```python
from build123d import *

# Parameters (mm, degrees)
SKETCH1_R           = 6.35
BOSS_EXTRUDE1_DEPTH = 3.175
SKETCH2_W           = 5.08
SKETCH2_H           = 25.4
CUT_EXTRUDE1_DEPTH  = 7.35
SKETCH3_R           = 15.875
CUT_EXTRUDE2_DEPTH  = 7.35


with BuildPart() as part:
    # Sketch1 → Boss-Extrude1 (new body, symmetric)
    with BuildSketch(Plane.XY):
        with BuildLine():
            Line((-0.002676144, -12.7), (0.002676144, -12.7))
            Line((0.002676144, -12.7), (50.8, -12.7))
            ThreePointArc((50.8, -12.7), (71.550320151, -11.225320151), (73.025, 9.525))
            Line((73.025, 9.525), (73.025, 152.4))
            Line((73.025, 152.4), (-73.025, 152.4))
            Line((-73.025, 152.4), (-73.025, 9.525))
            ThreePointArc((-73.025, 9.525), (-71.550320151, -11.225320151), (-50.8, -12.7))
            Line((-50.8, -12.7), (-0.002676144, -12.7))
        make_face()
        with Locations((-60.325, 0)):
            Circle(SKETCH1_R, mode=Mode.SUBTRACT)
        with Locations((60.325, 0)):
            Circle(SKETCH1_R, mode=Mode.SUBTRACT)
    extrude(amount=BOSS_EXTRUDE1_DEPTH, both=True)

    # Sketch2 → Cut-Extrude1 (cut, through all)
    with BuildSketch(Plane.XY.offset(3.175)):
        with Locations((-45.593, 133.35)):
            Rectangle(SKETCH2_W, SKETCH2_H)
        with Locations((-45.593, 85.725)):
            Rectangle(SKETCH2_W, SKETCH2_H)
        with Locations((-45.593, 38.1)):
            Rectangle(SKETCH2_W, SKETCH2_H)
        with Locations((50.165, 133.35)):
            Rectangle(SKETCH2_W, SKETCH2_H)
        with Locations((50.165, 38.1)):
            Rectangle(SKETCH2_W, SKETCH2_H)
        with Locations((50.165, 85.725)):
            Rectangle(SKETCH2_W, SKETCH2_H)
    extrude(amount=-CUT_EXTRUDE1_DEPTH, mode=Mode.SUBTRACT)

    # Sketch3 → Cut-Extrude2 (cut, through all)
    with BuildSketch(Plane.XY.offset(3.175)):
        with Locations((9.525, -12.7)):
            Circle(SKETCH3_R)
    extrude(amount=-CUT_EXTRUDE2_DEPTH, mode=Mode.SUBTRACT)


solid = part.part
```
Part model, mm, in its own coordinate system. A direction names the side the tool comes from. Coordinates: 2 decimals unless noted, no trailing zeros. Loops run counter-clockwise (first coordinate to the right, second up) from the corner with the lowest first, then second, coordinate; pieces in that order, holes last. Notation, with made-up numbers: (-19.75, -10) - (-10.75, -10) arc R22 cw to (-10.75, 12) - close; hole circle Ø11 at (-27.75, 8.25). An arc over 180 degrees is marked (long way). Write item = value, one per line. Start each with the question number.
Item 1: Cut at C-C, the plane x = 60. Give the cut face in (y, z) (3 decimals), and give its area (3 significant figures).
Item 2: Cut at A-A, the plane y = 0. Give the cut face in (x, z) (3 decimals).
Item 3: Wall check: L1, parallel to X at y = 123, z = -1.5 (3 decimals); L2, parallel to X at y = 114.5, z = -0.25 (3 decimals); L3, parallel to Y at x = -34.5, z = 1.5. Give the ranges that are in metal, low to high. Write a range as from..to.
Item 4: Cut at B-B, the plane z = -2. State how many separate pieces and enclosed holes the cut face has, and give its area (3 significant figures).
Item 5: Cut at D-D, the plane y = 104.5. Give the cut face in (x, z) (3 decimals).
Item 6: 3-axis set-ups, long thin cutter, end or side, ignore diameter. For faces 1 (the flat face through (-29, -12.7, 0)), 2 (the flat face through (-1, 69, -3.175)), 3 (the flat face through (50, 98.425, 0)): which of +Z, -Z, +X, -X, +Y, -Y reach the whole face in a straight line?
Item 7: Flat gauge pins, fed straight in: pin 1 Ø1.9 at (y, z) = (130, 1.5) entering from +X (3 decimals); pin 2 Ø1.9 at (y, z) = (132, 1) entering from -X (3 decimals). Where does each tip first touch, or does it go through?
The answers:
q1.outline = (-15.872, -3.175) - (-6.342, -3.175) - (-6.342, 3.175) - (-15.872, 3.175) - close; (6.342, -3.175) - (152.4, -3.175) - (152.4, 3.175) - (6.342, 3.175) - close
q1.area = 988 mm2
q2.outline = (-76.2, -3.175) - (-66.675, -3.175) - (-66.675, 3.175) - (-76.2, 3.175) - close; (-53.975, -3.175) - (0, -3.175) - (0, 3.175) - (-53.975, 3.175) - close; (19.05, -3.175) - (53.975, -3.175) - (53.975, 3.175) - (19.05, 3.175) - close; (66.675, -3.175) - (76.2, -3.175) - (76.2, 3.175) - (66.675, 3.175) - close
q3.L1 = -73.025..-48.133, -43.053..47.625, 52.705..73.025
q3.L2 = -73.025..73.025
q3.L3 = -12.7..152.4
q4.separate_pieces = 1
q4.enclosed_holes = 8
q4.area = 22,800 mm2
q5.outline = (-73.025, -3.175) - (73.025, -3.175) - (73.025, 3.175) - (-73.025, 3.175) - close
q6.face_1 = +Z, -Z, -Y
q6.face_2 = -Z, +X, -X, +Y, -Y
q6.face_3 = +Z, -Z
q7.pin_1 = 73.025
q7.pin_2 = -73.025
